Model file for the job. Use its own axes, mm. Give positions to 0.01 mm unless a question says otherwise; leave off trailing zeros. Write each loop counter-clockwise with the first axis right and the second up, starting at its lowest first coordinate (ties: lowest second). Pieces come first, ordered by that corner, then holes. Notation, with made-up numbers: M 36,38 L 88,38 A19 ccw 88,58 Z; hole C -5,-15.75 d9. An arc over 180 degrees is marked long. Answer as a JSON object with one key per item and string values. Group by question number.
```python
from build123d import *

# Parameters (mm, degrees)
SKETCH1_R           = 1.5
BOSS_EXTRUDE1_DEPTH = 4


with BuildPart() as part:
    # Sketch1 → Boss-Extrude1 (new body)
    # profile 1 of 2: a face of its own
    with BuildSketch(Plane.XY):
        with BuildLine():
            Line((0, 43.02618472), (-22, 43.02618472))
            Line((-22, 43.02618472), (-34.124535685, 43.02618472))
            ThreePointArc((-34.124535685, 43.02618472), (-35.892302638, 42.293951673), (-36.624535685, 40.52618472))
            ThreePointArc((-36.624535685, 40.52618472), (-35.892302638, 38.758417767), (-34.124535685, 38.02618472))
            ThreePointArc((-34.124535685, 38.02618472), (-28.821234826, 35.829485579), (-26.624535685, 30.52618472))
            Line((-26.624535685, 30.52618472), (-26.624535685, -6.97381528))
            ThreePointArc((-26.624535685, -6.97381528), (-29.02618472, -13.624535685), (-22.375464315, -16.02618472))
            Line((-22.375464315, -16.02618472), (-22.205082013, -15.942223704))
            Line((-22.205082013, -15.942223704), (-4.420251148, -7.178212035))
            ThreePointArc((-4.420251148, -7.178212035), (0, -6.148238779), (4.420251148, -7.178212035))
            Line((4.420251148, -7.178212035), (22.205082013, -15.942223704))
            Line((22.205082013, -15.942223704), (22.375464315, -16.02618472))
            ThreePointArc((22.375464315, -16.02618472), (29.02618472, -13.624535685), (26.624535685, -6.97381528))
            Line((26.624535685, -6.97381528), (26.624535685, 30.52618472))
            ThreePointArc((26.624535685, 30.52618472), (28.821234826, 35.829485579), (34.124535685, 38.02618472))
            ThreePointArc((34.124535685, 38.02618472), (35.892302638, 38.758417767), (36.624535685, 40.52618472))
            ThreePointArc((36.624535685, 40.52618472), (35.892302638, 42.293951673), (34.124535685, 43.02618472))
            Line((34.124535685, 43.02618472), (22, 43.02618472))
            Line((22, 43.02618472), (0, 43.02618472))
        make_face()
        with Locations((-24.5, -11.5)):
            Circle(SKETCH1_R, mode=Mode.SUBTRACT)
        Circle(SKETCH1_R, mode=Mode.SUBTRACT)
        with Locations((24.5, -11.5)):
            Circle(SKETCH1_R, mode=Mode.SUBTRACT)
        with BuildLine():
            Line((14.374535685, -1.22381528), (2.124535685, 4.52618472))
            ThreePointArc((2.124535685, 4.52618472), (0, 5), (-2.124535685, 4.52618472))
            Line((-2.124535685, 4.52618472), (-14.374535685, -1.22381528))
            Line((-14.374535685, -1.22381528), (-2.097868645, 10.785812849))
            ThreePointArc((-2.097868645, 10.785812849), (0, 11.641297251), (2.097868645, 10.785812849))
            Line((2.097868645, 10.785812849), (14.374535685, -1.22381528))
        make_face(mode=Mode.SUBTRACT)
        with BuildLine():
            Line((-6.73171968, 15.226590291), (-19.124535685, 2.558215038))
            Line((-19.124535685, 2.558215038), (-19.124535685, 31.546592884))
            Line((-19.124535685, 31.546592884), (-6.778366633, 19.468974534))
            ThreePointArc((-6.778366633, 19.468974534), (-5.876416612, 17.357443313), (-6.73171968, 15.226590291))
        make_face(mode=Mode.SUBTRACT)
        with Locations((-34.124535685, 40.52618472)):
            Circle(SKETCH1_R, mode=Mode.SUBTRACT)
        with BuildLine():
            Line((-1.833941699, 24.523340745), (-14.124535685, 36.546592884))
            Line((-14.124535685, 36.546592884), (14.124535685, 36.546592884))
            Line((14.124535685, 36.546592884), (2.408442543, 24.569987698))
            ThreePointArc((2.408442543, 24.569987698), (0.296911322, 23.668037677), (-1.833941699, 24.523340745))
        make_face(mode=Mode.SUBTRACT)
        with Locations((-14.124535685, 40.02618472)):
            Circle(SKETCH1_R, mode=Mode.SUBTRACT)
        with BuildLine():
            Line((19.124535685, 31.546592884), (19.124535685, 4.020746784))
            Line((19.124535685, 4.020746784), (7.24778827, 15.639154236))
            ThreePointArc((7.24778827, 15.639154236), (6.345656915, 17.783669834), (7.24778827, 19.928185432))
            Line((7.24778827, 19.928185432), (19.124535685, 31.546592884))
        make_face(mode=Mode.SUBTRACT)
        with Locations((14.124535685, 40.02618472)):
            Circle(SKETCH1_R, mode=Mode.SUBTRACT)
        with Locations((34.124535685, 40.52618472)):
            Circle(SKETCH1_R, mode=Mode.SUBTRACT)
    # profile 2 of 2: a face of its own
    with BuildSketch(Plane.XY):
        with BuildLine():
            Line((-34.124535685, 43.02618472), (-22, 43.02618472))
            Line((-22, 43.02618472), (0, 43.02618472))
            Line((0, 43.02618472), (22, 43.02618472))
            Line((22, 43.02618472), (34.124535685, 43.02618472))
            ThreePointArc((34.124535685, 43.02618472), (35.892302638, 42.293951673), (36.624535685, 40.52618472))
            Line((36.624535685, 40.52618472), (36.624535685, 45.02618472))
            Line((36.624535685, 45.02618472), (-36.624535685, 45.02618472))
            Line((-36.624535685, 45.02618472), (-36.624535685, 40.52618472))
            ThreePointArc((-36.624535685, 40.52618472), (-35.892302638, 42.293951673), (-34.124535685, 43.02618472))
        make_face()
    extrude(amount=BOSS_EXTRUDE1_DEPTH)


solid = part.part
```
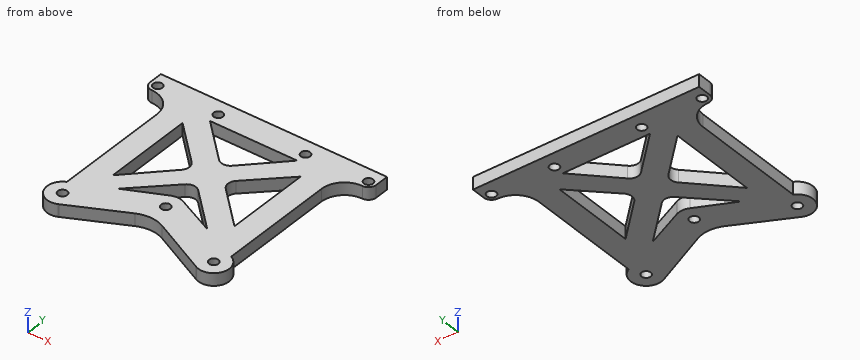
Q1. Slice it at D-D, the plane x = 16.5. Write the cut outline in (y, z), then the cut area to 3 significant figures.
Q2. Slice it at B-B, the plane y = -11.5. Write the cut outline in (x, z), then the cut area to 3 significant figures.
Q3. Slice it at A-A, the plane x = -24.5. Write the cut outline in (y, z).
Q4. Slice it at C-C, the plane x = 0. Write the cut outline in (y, z).
Q5. Wall check: L1, parallel to X at y = -11, z = 0.45; L2, parallel to X at y = 14.5, z = 0.65; L3, parallel to Y at x = 24.5, z = 2.05. Give the ranges that are in metal, low to high.
Q6. Drop flat-ended pins along their axis: P1, Ø1.5, axis at y = 26.5, z = 3, coming from the +X side; P2, Ø1.2, axis at y = 18, z = 1.5, coming from the -X side; P3, Ø2, axis at x = 5, z = 3.5, coming from the -Y side. Give the stop position or say it passes through.
Solved:
{
 "1": {"outline": "M -13.13,0 L 6.59,0 L 6.59,4 L -13.13,4 Z; M 28.98,0 L 45.03,0 L 45.03,4 L 28.98,4 Z", "area": "143 mm²"},
 "2": {"outline": "M -29.5,0 L -26,0 L -26,4 L -29.5,4 Z; M -23,0 L -13.19,0 L -13.19,4 L -23,4 Z; M 13.19,0 L 23,0 L 23,4 L 13.19,4 Z; M 26,0 L 29.5,0 L 29.5,4 L 26,4 Z", "area": "106 mm²"},
 "3": {"outline": "M -16.5,0 L -13,0 L -13,4 L -16.5,4 Z; M -10,0 L 45.03,0 L 45.03,4 L -10,4 Z"},
 "4": {"outline": "M -6.15,0 L -1.5,0 L -1.5,4 L -6.15,4 Z; M 1.5,0 L 5,0 L 5,4 L 1.5,4 Z; M 11.64,0 L 23.68,0 L 23.68,4 L 11.64,4 Z; M 36.55,0 L 45.03,0 L 45.03,4 L 36.55,4 Z"},
 "5": {"L1": "x = -29.47 to -25.91, -23.09 to -12.18, 12.18 to 23.09, 25.91 to 29.47", "L2": "x = -26.62 to -19.12, -7.44 to 8.41, 19.12 to 26.62", "L3": "y = -16.5 to -13, -10 to 45.03"},
 "6": {"P1": "stops at x = 26.62", "P2": "stops at x = -26.62", "P3": "stops at y = -7.96"}
}
